CAD build for the part. Positions are in the model's coordinates, mm. Face numbers are marked on the shaded views. Give positions to 0.01 mm unless a question says otherwise; leave off trailing zeros. Order: outer loops, then holes, each group sorted by start corner. A loop starts at its lowest first (then second) coordinate and runs counter-clockwise, first axis right, second up.
Item 1: Two-plate mould, pull along Y, no slides. Class the marked faces 1, 2 and 3: released by +Y, released by -Y, zero draft, split by the parting line, or undercut.
Item 2: Band-saw the part on C-C on y = 15. Give the cut face in (x, z), plus the area to 3 significant figures.
Item 3: Band-saw the part on A-A on y = 20.25. Give the cut face in (x, z) (3 decimals).
Item 4: Band-saw the part on B-B on x = 16.75. Give the cut face in (y, z) (3 decimals), plus the area to 3 significant figures.
Item 5: Flat gauge pins, fed straight in: P1, Ø3, axis at x = 18, y = 15.5, coming from the -Z side; P2, Ø1.3, axis at y = 23.5, z = 0.5, coming from the -X side; P3, Ø1.3, axis at y = 25, z = 2, coming from the +X side; P4, Ø3, axis at x = 19, z = 12.5, coming from the -Y side. Where does each tip first touch, or does it go through?
Item 6: Wall check: L1, parallel to Y at x = 16, z = 13.5; L2, parallel to Z at x = 14.25, y = 24.5 (3 decimals); L3, parallel to X at y = 20.5, z = 8.5. Give the ranges that are in metal, low to high.
Item 7: Band-saw the part on D-D on x = 18.25. Give the cut face in (y, z) (3 decimals).
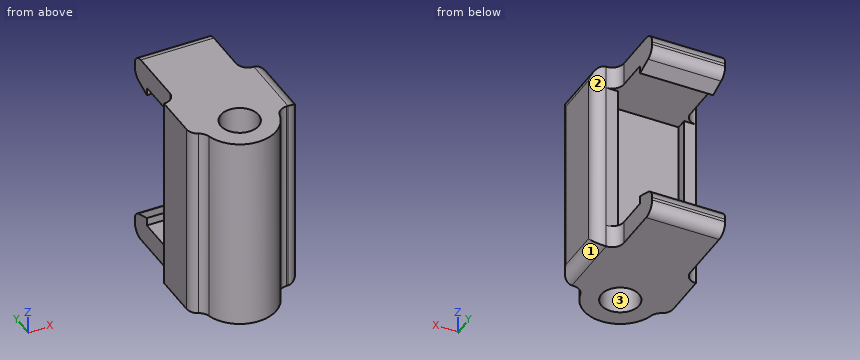
```python
from build123d import *

# Parameters (mm, degrees)
ESBO_O1_R                = 3.1
ESBO_O1_R_2              = 1.55
RESSALTO_EXTRUS_O1_DEPTH = 16.74
BOSS_EXTRUDE1_DEPTH      = 16.74
SKETCH2_W                = 6.2
SKETCH2_H                = 1.955
BOSS_EXTRUDE2_DEPTH      = 7.715
BOSS_EXTRUDE3_DEPTH      = 6.2
SKETCH5_W                = 16.74
SKETCH5_H                = 5.66650546
BOSS_EXTRUDE4_DEPTH      = 2
SKETCH6_W                = 16.74
SKETCH6_H                = 4.529470895
BOSS_EXTRUDE5_DEPTH      = 1
FILLET1_R                = 1
FILLET4_R                = 1
M3_CLEARANCE_HOLE1_D     = 3.2


with BuildPart() as part:
    # Esboço1 → Ressalto-extrusão1 (new body)
    with BuildSketch(Plane.XY):
        with Locations((16.016666667, 16.016666667)):
            Circle(ESBO_O1_R)
        with Locations((16.016666667, 16.016666667)):
            Circle(ESBO_O1_R_2, mode=Mode.SUBTRACT)
    extrude(amount=RESSALTO_EXTRUS_O1_DEPTH)

    # Sketch1 → Boss-Extrude1 (add)
    with BuildSketch(Plane(origin=(0, 0, 0), x_dir=(-1, 0, 0), z_dir=(0, 0, -1))):
        with BuildLine():
            Line((-12.916666667, 16.016666667), (-12.916666667, 19.634677588))
            Line((-12.916666667, 19.634677588), (-19.116666667, 19.634677588))
            Line((-19.116666667, 19.634677588), (-19.116666667, 16.016666667))
            ThreePointArc((-19.116666667, 16.016666667), (-16.016666667, 19.116666667), (-12.916666667, 16.016666667))
        make_face()
    extrude(amount=-BOSS_EXTRUDE1_DEPTH)

    # Sketch2 → Boss-Extrude2 (add)
    with BuildSketch(Plane(origin=(0, 19.634677588, 0), x_dir=(1, 0, 0), z_dir=(0, 1, 0))):
        with Locations((16.016666667, -0.9775)):
            Rectangle(SKETCH2_W, SKETCH2_H)
        with Locations((16.016666667, -15.7625)):
            Rectangle(SKETCH2_W, SKETCH2_H)
    extrude(amount=BOSS_EXTRUDE2_DEPTH)

    # Sketch4 → Boss-Extrude3 (add)
    with BuildSketch(Plane.ZY.offset(-12.916666667)):
        Polygon((1.955, 27.349677588), (1.955, 25.349677588), (2.639300497, 25.349677588), align=None)
        Polygon((14.100699503, 25.349677588), (14.785, 27.349677588), (14.785, 25.349677588), align=None)
    extrude(amount=-BOSS_EXTRUDE3_DEPTH)

    # Sketch5 → Boss-Extrude4 (add)
    with BuildSketch(Plane(origin=(19.116666667, 0, 0), x_dir=(0, 0, -1), z_dir=(1, 0, 0))):
        with Locations((-8.37, 18.849919397)):
            Rectangle(SKETCH5_W, SKETCH5_H)
    extrude(amount=BOSS_EXTRUDE4_DEPTH)

    # Sketch6 → Boss-Extrude5 (add)
    with BuildSketch(Plane.ZY.offset(-12.916666667)):
        with Locations((8.37, 18.281402115)):
            Rectangle(SKETCH6_W, SKETCH6_H)
    extrude(amount=BOSS_EXTRUDE5_DEPTH)

    # Fillet1
    fillet1_edges = [part.edges().sort_by_distance(p)[0] for p in [
        (21.116666667, 21.683172127, 8.37),
        (21.116666667, 18.849919397, 0),
        (21.116666667, 16.016666667, 8.37),
        (21.116666667, 18.849919397, 16.74),
        (16.016666667, 27.349677588, 0),
        (16.016666667, 27.349677588, 1.955),
        (16.016666667, 27.349677588, 16.74),
        (16.016666667, 27.349677588, 14.785),
        (19.116666667, 21.683172127, 15.7625),
        (12.916666667, 20.546137562, 15.7625),
        (12.916666667, 20.546137562, 0.9775),
        (19.116666667, 21.683172127, 0.9775),
        (12.916666667, 16.016666667, 8.37),
        (19.116666667, 16.016666667, 8.37),
    ]]
    fillet(fillet1_edges, radius=FILLET1_R - 0.0001)  # a hair under: the kernel refuses the full size

    # Fillet4
    fillet4_edges = [part.edges().sort_by_distance(p)[0] for p in [
        (11.916666667, 16.016666667, 8.37),
    ]]
    fillet(fillet4_edges, radius=FILLET4_R)

    # M3 Clearance Hole1 (through all)
    with Locations(Plane(origin=(0, 0, 0), x_dir=(-1, 0, 0), z_dir=(0, 0, -1))):
        with Locations((-16.016666667, 16.016666667)):
            Hole(M3_CLEARANCE_HOLE1_D / 2)


solid = part.part
```
The answers:
1. face 1: zero draft
1. face 2: released by +Y
1. face 3: undercut
2. outline: (13.09, 0) - (14.78, 0) - (14.78, 16.74) - (13.09, 16.74) - close; (17.25, 0) - (18.95, 0) - (18.95, 16.74) - (17.25, 16.74) - close
2. area: 56.7 mm2
3. outline: (11.917, 0) - (20.117, 0) arc R1 ccw to (21.117, 1) - (21.117, 15.74) arc R1 ccw to (20.117, 16.74) - (11.917, 16.74) - close; hole (12.917, 1.955) - (19.117, 1.955) - (19.117, 14.785) - (12.917, 14.785) - close
4. outline: (13.005, 0) - (14.595, 0) - (14.595, 16.74) - (13.005, 16.74) - close; (17.439, 0) - (26.35, 0) arc R1 ccw to (27.35, 1) - (27.35, 1.24) arc R1 ccw to (26.673, 2.186) - (25.35, 2.639) - (25.35, 1.955) - (19.635, 1.955) - (19.635, 14.785) - (25.35, 14.785) - (25.35, 14.101) - (26.673, 14.554) arc R1 ccw to (27.35, 15.5) - (27.35, 15.74) arc R1 ccw to (26.35, 16.74) - (17.439, 16.74) - close
4. area: 94.3 mm2
5. P1: stops at z = 0
5. P2: stops at x = 12.92
5. P3: stops at x = 19.12
5. P4: stops at y = 13.29
6. L1: y = 12.92 to 14.42, 17.62 to 19.63
6. L2: z = 0 to 1.955, 14.785 to 16.74
6. L3: x = 11.92 to 12.92, 19.12 to 21.12
7. outline: (13.867, 0) - (26.35, 0) arc R1 ccw to (27.35, 1) - (27.35, 1.24) arc R1 ccw to (26.673, 2.186) - (25.35, 2.639) - (25.35, 1.955) - (19.635, 1.955) - (19.635, 14.785) - (25.35, 14.785) - (25.35, 14.101) - (26.673, 14.554) arc R1 ccw to (27.35, 15.5) - (27.35, 15.74) arc R1 ccw to (26.35, 16.74) - (13.867, 16.74) - close
